from build123d import *

# Parameters (mm, degrees)
BOSS_EXTRUDE1_DEPTH       = 55
TOP_TAB_NOTCH_REACH       = 197.475
BOTTOM_TAB_NOTCH_REACH    = 197.475
BOTTOM_CENTER_SLOTS_REACH = 197.475
SKETCH6_W                 = 3.4
SKETCH6_H                 = 10.641777725


with BuildPart() as part:
    # Sketch1 → Boss-Extrude1 (new, symmetric)
    with BuildSketch(Plane.XY):
        Polygon((-44.702851081, 214.841310922), (-71.856111855, 140.238340079), (-69.037033993, 139.212279649), (-41.883773219, 213.815250492), align=None)
    extrude(amount=BOSS_EXTRUDE1_DEPTH, both=True)

    # Sketch3 → top tab notch (cut, up to next)
    with BuildSketch(Plane(origin=(-108.522277226, 39.498878665, 0), x_dir=(0, 0, 1), z_dir=(-0.9396926207859095, 0.34202014332566577, 0)), mode=Mode.PRIVATE) as top_tab_notch_sk1:
        with BuildLine():
            Line((47, 186.595518979), (-47, 186.595518979))
            Line((-47, 186.595518979), (-47, 185.462807478))
            ThreePointArc((-47, 185.462807478), (-46.6, 184.712807478), (-47, 183.962807478))
            Line((-47, 183.962807478), (-47, 179.678363458))
            Line((-47, 179.678363458), (-42, 179.678363458))
            Line((-42, 179.678363458), (-42, 174.678363458))
            Line((-42, 174.678363458), (-47, 174.678363458))
            Line((-47, 174.678363458), (-47, 168.728030606))
            Line((-47, 168.728030606), (-14.1, 168.728030606))
            Line((-14.1, 168.728030606), (-14.1, 144.678363458))
            Line((-14.1, 144.678363458), (-9, 144.678363458))
            Line((-9, 144.678363458), (-9, 168.728030606))
            Line((-9, 168.728030606), (9, 168.728030606))
            Line((9, 168.728030606), (9, 144.678363458))
            Line((9, 144.678363458), (14.1, 144.678363458))
            Line((14.1, 144.678363458), (14.1, 168.728030606))
            Line((14.1, 168.728030606), (47, 168.728030606))
            Line((47, 168.728030606), (47, 174.678363458))
            Line((47, 174.678363458), (42, 174.678363458))
            Line((42, 174.678363458), (42, 179.678363458))
            Line((42, 179.678363458), (47, 179.678363458))
            Line((47, 179.678363458), (47, 183.962807478))
            ThreePointArc((47, 183.962807478), (46.6, 184.712807478), (47, 185.462807478))
            Line((47, 185.462807478), (47, 186.595518979))
        make_face()
    top_tab_notch_tool1 = extrude(top_tab_notch_sk1.sketch, amount=-TOP_TAB_NOTCH_REACH, mode=Mode.PRIVATE) & part.part
    add(top_tab_notch_tool1.solids().sort_by_distance((-48.693367, 203.877457, 0))[0], mode=Mode.SUBTRACT)

    # Sketch5 → bottom tab notch (cut, up to next)
    with BuildSketch(Plane(origin=(-108.522277226, 39.498878665, 0), x_dir=(0, 0, 1), z_dir=(-0.9396926207859096, 0.34202014332566527, 0)), mode=Mode.PRIVATE) as bottom_tab_notch_sk1:
        with BuildLine():
            Line((47, 107.204695648), (47, 108.337407149))
            ThreePointArc((47, 108.337407149), (46.6, 109.087407149), (47, 109.837407149))
            Line((47, 109.837407149), (47, 114.121851169))
            Line((47, 114.121851169), (-47, 114.121851169))
            Line((-47, 114.121851169), (-47, 109.837407149))
            ThreePointArc((-47, 109.837407149), (-46.6, 109.087407149), (-47, 108.337407149))
            Line((-47, 108.337407149), (-47, 107.204695648))
            Line((-47, 107.204695648), (47, 107.204695648))
        make_face()
    bottom_tab_notch_tool1 = extrude(bottom_tab_notch_sk1.sketch, amount=-BOTTOM_TAB_NOTCH_REACH, mode=Mode.PRIVATE) & part.part
    add(bottom_tab_notch_tool1.solids().sort_by_distance((-70.672508, 143.490264, 0))[0], mode=Mode.SUBTRACT)

    # Sketch6 → bottom center slots (cut, up to next)
    with BuildSketch(Plane(origin=(-108.522277226, 39.498878665, 0), x_dir=(0, 0, 1), z_dir=(-0.9396926207859096, 0.34202014332566527, 0)), mode=Mode.PRIVATE) as bottom_center_slots_sk1:
        with Locations((8.5, 119.442740032)):
            Rectangle(SKETCH6_W, SKETCH6_H)
    bottom_center_slots_tool1 = extrude(bottom_center_slots_sk1.sketch, amount=-BOTTOM_CENTER_SLOTS_REACH, mode=Mode.PRIVATE) & part.part
    # Sketch6 → bottom center slots (cut, up to next)
    with BuildSketch(Plane(origin=(-108.522277226, 39.498878665, 0), x_dir=(0, 0, 1), z_dir=(-0.9396926207859096, 0.34202014332566527, 0)), mode=Mode.PRIVATE) as bottom_center_slots_sk2:
        with Locations((-8.5, 119.442740032)):
            Rectangle(SKETCH6_W, SKETCH6_H)
    bottom_center_slots_tool2 = extrude(bottom_center_slots_sk2.sketch, amount=-BOTTOM_CENTER_SLOTS_REACH, mode=Mode.PRIVATE) & part.part
    add(bottom_center_slots_tool1.solids().sort_by_distance((-67.670454, 151.73834, 8.5))[0], mode=Mode.SUBTRACT)
    add(bottom_center_slots_tool2.solids().sort_by_distance((-67.670454, 151.73834, -8.5))[0], mode=Mode.SUBTRACT)


solid = part.part
Model file for the job. Use its own axes, mm. A direction names the side the tool comes from. Coordinates: 2 decimals unless noted, no trailing zeros. Loops run counter-clockwise (first coordinate to the right, second up) from the corner with the lowest first, then second, coordinate; pieces in that order, holes last. Notation, with made-up numbers: (5.25, -38) -> (45.25, -38) arc R35 cw to (45.25, -5) -> close; hole circle Ø4 at (-13, 55). An arc over 180 degrees is marked (long way). Use one line per item in the form item = value. Start each with the question number.
(1) Cut at A-A on y = 154.5. Give the cut face in (x, z).
(2) Cut at B-B on x = -57.75. Give the cut face in (y, z).
(3) Pull direction Z, two halves, no side cores. Call faces 1 (the flat face through (-57, 177, 55)), 2 (the flat face through (-47.389, 203.137, 44.535)), 3 (the flat face through (-70.466, 139.732, -50.944)): pulls with the +Z half, pulls with the -Z half, needs draft (parallel to the pull), parting line crosses it, or undercut.
(4) Flat gauge pins, fed straight in: pin 1 (3 mm diameter, centred on x = -65, y = 150, fed in from +Z); pin 2 (8 mm diameter, centred on y = 168.5, z = -43.5, fed in from -X). Where does each tip first touch, or does it go through?
(5) Cut at C-C on z = 4. Give the cut face in (x, y), and give its area (3 significant figures).
(6) Cut at D-D on y = 181. Give the cut face in (x, z), and give its area (3 significant figures).
(7) Tool access for faces 4 (the flat face through (-70, 140, -47)), 5 (the flat face through (-47.389, 203.137, -44.465)), 6 (the flat face through (-70.466, 139.732, 51.056)), 7 (the flat face through (-69, 144, -47)): list every direction of +Z, -Z, +X, -X, +Y, -Y with a clear straight run to the whole face (end or side of a thin tool).
(8) Probe probe 1 along Z at (x, y) = (-48.25, 201); probe 2 along X at (y, z) = (181.5, 36); probe 3 along X at (y, z) = (147.5, 5). List the from-to ranges inside material, lowest first. Write a range as from..to.
Values:
q1.outline = (-66.67, -55) -> (-63.47, -55) -> (-63.47, -10.2) -> (-66.67, -10.2) -> close; (-66.67, -6.8) -> (-63.47, -6.8) -> (-63.47, 6.8) -> (-66.67, 6.8) -> close; (-66.67, 10.2) -> (-63.47, 10.2) -> (-63.47, 55) -> (-66.67, 55) -> close
q2.outline = (170.22, -55) -> (178.99, -55) -> (178.99, -14.1) -> (174.98, -14.1) -> (174.98, -9) -> (178.99, -9) -> (178.99, 9) -> (174.98, 9) -> (174.98, 14.1) -> (178.99, 14.1) -> (178.99, 55) -> (170.22, 55) -> close
q3.face_1 = pulls with the +Z half
q3.face_2 = undercut
q3.face_3 = needs draft
q4.pin_1 = 55
q4.pin_2 = -63.03
q5.outline = (-69.49, 146.74) -> (-66.67, 145.71) -> (-47.99, 197.03) -> (-50.81, 198.05) -> close
q5.area = 164 mm2
q6.outline = (-57.02, -55) -> (-53.83, -55) -> (-53.83, -14.1) -> (-57.02, -14.1) -> close; (-57.02, -9) -> (-53.83, -9) -> (-53.83, 9) -> (-57.02, 9) -> close; (-57.02, 14.1) -> (-53.83, 14.1) -> (-53.83, 55) -> (-57.02, 55) -> close
q6.area = 319 mm2
q7.face_4 = -X, -Y
q7.face_5 = -X
q7.face_6 = +Z, -Z, -X, -Y
q7.face_7 = none
q8.probe_1 = -55..-47, 47..55
q8.probe_2 = -56.84..-53.65
q8.probe_3 = -69.21..-66.02
